```python
from build123d import *

# Parameters (mm, degrees)
BOSS_EXTRUDE1_DEPTH = 1.5875
FILLET1_R           = 0.635


with BuildPart() as part:
    # Sketch1 → Boss-Extrude1 (new, symmetric)
    with BuildSketch(Plane.XY):
        Polygon((0, 0), (0, 6.604), (3.175, 6.604), (50.8, 3.175), (50.8, 0), align=None)
    extrude(amount=BOSS_EXTRUDE1_DEPTH, both=True)

    # Fillet1
    fillet1_edges = [part.edges().sort_by_distance(p)[0] for p in [
        (50.8, 3.175, 0),
    ]]
    fillet(fillet1_edges, radius=FILLET1_R)


solid = part.part
```
Verification items for the finished model (mm, model axes). Coordinates: 2 decimals unless noted, no trailing zeros. Write each loop counter-clockwise with the first axis right and the second up, starting at its lowest first coordinate (ties: lowest second). Pieces come first, ordered by that corner, then holes. Notation, with made-up numbers: (-2, 26) - (14, 26) arc R16 ccw to (14, 48) - close; hole circle Ø4 at (77, 68). An arc over 180 degrees is marked (long way). One line per question, with ' | ' between items. Start each with the question number.
1. Section check B-B (x = 42). Enter the section's corners in (y, z).
2. Section check A-A (z = -0.6). Enter the section's corners in (x, y) (3 decimals), plus the area to 3 significant figures.
3. Gauge pin test, flat ends, axial feed: P1, Ø1.5, axis at y = 5.5, z = -1, coming from the -X side; P2, Ø1.5, axis at x = 19, z = -0.5, coming from the +Y side. Record the tip position at first contact, or that the pin passes through.
4. Material ranges on line 1 along Y through (x, z) = (21.5, 1.05); line 2 along Y through (x, z) = (34, -0.45), recorded low to high.
5. Section check C-C (y = 6). Enter the section's corners in (x, z).
Computed values:
1) outline: (0, -1.59) - (3.81, -1.59) - (3.81, 1.59) - (0, 1.59) - close
2) outline: (0, 0) - (50.8, 0) - (50.8, 2.584) arc R0.635 ccw to (50.211, 3.217) - (3.175, 6.604) - (0, 6.604) - close | area: 254 mm²
3) P1: x = 0 | P2: y = 5.52
4) line 1: 0 to 5.28 | line 2: 0 to 4.38
5) outline: (0, -1.59) - (11.56, -1.59) - (11.56, 1.59) - (0, 1.59) - close
